Input: part model. Units: mm. Frame: model coordinates. Give positions to 0.01 mm unless a question says otherwise; leave off trailing zeros. Order: outer loops, then holes, each group sorted by start corner. A loop starts at its lowest first (then second) coordinate and runs counter-clockwise, first axis right, second up. Notation, with made-up numbers: (63.25, 84.5) - (79.25, 84.5) arc R38 ccw to (79.25, 122.5) - close; hole circle Ø10 at (51.25, 73). An arc over 180 degrees is marked (long way). Answer in a Markdown table with one row per item. Add a question column.
1. Mould query, pull axis Y, two halves, no side actions, for faces 1 (the face through (0, 0, -2.75)), 2 (the face through (-1.104, -1.46, -2.525)), 3 (the face through (0.013, -0.976, -0.748)), 4 (the face through (-0.02, 2.39, 1.36)). Classes: released by +Y, released by -Y, zero draft, split by the parting line, or undercut.
2. Ray query, line 1 (Z direction, x = -0.1, y = 0); line 2 (Z direction, x = 1, y = 1); line 3 (Y direction, x = 0.75, z = -0.25). Return the intervals inside material, ascending. Write a range as [from, to].
3. Section query A-A on x = 0.8. Return loops of the section in (y, z), and give its area (3 significant figures).
Autodesk Inventor part; units mm, degrees
ref_plane "cp_XY" through (1.2, 0, 0) normal (1, 0, 0) x (0, 0, -1)
ref_plane "cp_YZ" through (1.2, 0, 0) normal (0, 0, -1) x (0, 1, 0)
ref_plane "cp_ZX" through (1.2, 0, 0) normal (0, 1, 0) x (1, 0, 0)
sketch "Sketch_1" plane through (0, 0, 0) normal (0, 0, 1) x (1, 0, 0)
  line L0 (1.2, 0) -> (-1.2, 0)
  line L1 (-1.2, 0) -> (-1.2, 2.75)
  line L2 (-1.2, 2.75) -> (-0.9402, 3.2)
  line L3 (-0.9402, 3.2) -> (1.2, 3.2)
  line L4 (1.2, 3.2) -> (1.2, 0)
  line L5 (1.2, 0) -> (-1.2, 0)
revolve "Revolution1" add sketch "Sketch_1" angle 360 about axis through (1.2, 0, 0) along (1, 0, 0)
sketch "Sketch_2" plane through (0, 0, 0) normal (0, 0, 1) x (1, 0, 0)
  line L0 (1.2, 0) -> (-1.2, 0)
  line L1 (-1.2, 0) -> (-1.2, 1.5)
  line L2 (-1.2, 1.5) -> (-0.9295, 1.2295)
  line L3 (-0.9295, 1.2295) -> (0.9295, 1.2295)
  line L4 (0.9295, 1.2295) -> (1.2, 1.5)
  line L5 (1.2, 1.5) -> (1.2, 0)
  line L6 (1.2, 0) -> (-1.2, 0)
revolve "Revolution2" cut sketch "Sketch_2" angle 360 about axis through (1.2, 0, 0) along (1, 0, 0)
thread "Thread1"
sketch "Sketch_3" plane through (0, 0, 0) normal (1, 0, 0) x (0, 1, 0)
  line L0 (-5.5, 5.5) -> (-5.5, -5.5)
  line L1 (-5.5, -5.5) -> (5.5, -5.5)
  line L2 (5.5, -5.5) -> (5.5, 5.5)
  line L3 (5.5, 5.5) -> (-5.5, 5.5)
  line L4 (-1.5877, 2.75) -> (-3.1754, 0)
  line L5 (-3.1754, 0) -> (-1.5877, -2.75)
  line L6 (-1.5877, -2.75) -> (1.5877, -2.75)
  line L7 (1.5877, -2.75) -> (3.1754, 0)
  line L8 (3.1754, 0) -> (1.5877, 2.75)
  line L9 (1.5877, 2.75) -> (-1.5877, 2.75)
extrude "Extrusion1" cut sketch "Sketch_3" along normal mid plane 2.4
ref_plane "cp_XY" through (1.2, 0, 0) normal (1, 0, 0) x (0, 0, -1)
ref_plane "cp_YZ" through (1.2, 0, 0) normal (0, 0, -1) x (0, 1, 0)
ref_plane "cp_ZX" through (1.2, 0, 0) normal (0, 1, 0) x (1, 0, 0)
ref_plane "nut_to_screw_XY" through (0, 0, 0) normal (1, 0, 0) x (0, 0, -1)
ref_plane "nut_to_screw_YZ" through (0, 0, 0) normal (0, 0, -1) x (0, 1, 0)
ref_plane "nut_to_screw_ZX" through (0, 0, 0) normal (0, 1, 0) x (1, 0, 0)
properties part number "LBNR3" material "鋼、炭素鋼"
Answer:
| question | item | result |
|---|---|---|
| 1 | face 1 | zero draft |
| 1 | face 2 | released by -Y |
| 1 | face 3 | undercut |
| 1 | face 4 | released by +Y |
| 2 | line 1 | z = [-2.75, -1.23], [1.23, 2.75] |
| 2 | line 2 | z = [-2.75, -0.83], [0.83, 2.75] |
| 2 | line 3 | y = [-3.03, -1.2], [1.2, 3.03] |
| 3 | outline | (-3.18, 0) - (-1.59, -2.75) - (1.59, -2.75) - (3.18, 0) - (1.59, 2.75) - (-1.59, 2.75) - close; hole circle Ø2.46 at (0, 0) |
| 3 | area | 21.4 mm² |
